```python
from build123d import *

# Parameters (mm, degrees)
F0_W     = 152.893602
F0_H     = 101.389184
F1_DEPTH = 24.13
F2_T     = -12.7
F3_R     = 3.028448
F3_R_2   = 3.005177
F4_DEPTH = 101.389185


with BuildPart() as f1:
    # F0 (on Top) → F1 (new body)
    with BuildSketch(Plane.XY):
        Rectangle(F0_W, F0_H)
    extrude(amount=F1_DEPTH)

    # F2
    f2_openings = [f1.faces().sort_by_distance(p)[0] for p in [
        (0, 0, 24.13),
    ]]
    offset(amount=F2_T, openings=f2_openings)

    # F3 (on face) → F4 (cut, through all)
    with BuildSketch(Plane(origin=(0, 50.694592, 0), x_dir=(-1, 0, 0), z_dir=(0, 1, 0))):
        with Locations((-63.746801, 12.7)):
            Circle(F3_R)
        with Locations((63.746801, 12.7)):
            Circle(F3_R_2)
    extrude(amount=-F4_DEPTH, mode=Mode.SUBTRACT)


solid = f1.part
```
Build history of the part. All positions in model axes, mm. A direction names the side the tool comes from. Give positions to 0.01 mm unless a question says otherwise; leave off trailing zeros. Loops run counter-clockwise (first coordinate to the right, second up) from the corner with the lowest first, then second, coordinate; pieces in that order, holes last. Notation, with made-up numbers: (86, 39.5) - (108, 39.5) arc R32 cw to (108, 66.5) - close; hole circle Ø9 at (60, 5.5). An arc over 180 degrees is marked (long way). Use a Markdown table: item, result.
(1) Drop a flat-ended pin along its axis: pin 1 Ø23 at (x, y) = (-26.5, -6.5) entering from +Z. Give the stop position or say it passes through.
Taken from the geometry:
| item | result |
|---|---|
| pin 1 | z = 12.7 |
(2) Which spindle directions (+Z, -Z, +X, -X, +Y, -Y) get a long thin tool onto all of the face, cutting with end or side? Do faces 4 (the face through (-1, 50.695, 12)), 5 (the face through (63.747, -1, 20)). Say none if no direction does.
Taken from the geometry:
| item | result |
|---|---|
| face 4 | +Z, -Z, +X, -X, +Y |
| face 5 | +Z |
(3) Wall check: line 1 along X through (y, z) = (-41, 15.25); line 2 along Y through (x, z) = (-55, 20.5); line 3 along X through (y, z) = (-36, 20.75). Give the ranges that are in metal, low to high.
Taken from the geometry:
| item | result |
|---|---|
| line 1 | -76.45 to -65.34, -62.16 to 62.11, 65.38 to 76.45 |
| line 2 | -50.69 to -37.99, 37.99 to 50.69 |
| line 3 | -76.45 to -63.75, 63.75 to 76.45 |
(4) Band-saw the part on A-A (y = -41.5). Give the cut face in (x, z).
Taken from the geometry:
| item | result |
|---|---|
| outline | (-76.45, 0) - (76.45, 0) - (76.45, 24.13) - (-76.45, 24.13) - close; hole circle Ø6.01 at (-63.75, 12.7); hole circle Ø6.06 at (63.75, 12.7) |
(5) Pull direction Z, two halves, no side cores. Call faces 1 (the face through (-76.447, -1, 12)), 2 (the face through (-1, 1, 0)), 3 (the face through (-66.5, 0.7, 11.5)): +Z half, -Z half, draft (parallel to the pull), parting line (faces both ways), or undercut.
Taken from the geometry:
| item | result |
|---|---|
| face 1 | draft |
| face 2 | -Z half |
| face 3 | undercut |
(6) Band-saw the part on B-B (x = -52.5). Give the cut face in (y, z), and give its area (3 significant figures).
Taken from the geometry:
| item | result |
|---|---|
| outline | (-50.69, 0) - (50.69, 0) - (50.69, 24.13) - (37.99, 24.13) - (37.99, 12.7) - (-37.99, 12.7) - (-37.99, 24.13) - (-50.69, 24.13) - close |
| area | 1,580 mm2 |
